from build123d import *

# Parameters (mm, degrees)
F1_DEPTH = 32
F2_R     = 6.5
F3_DEPTH = 25
F4_R     = 6.5
F5_DEPTH = 25
F6_R     = 6.5
F7_DEPTH = 25
F8_R     = 6.5
F9_DEPTH = 25


with BuildPart() as f1:
    # F0 (on Front) → F1 (new body)
    with BuildSketch(Plane.XZ):
        Polygon((0, 19.488953), (0, 0), (44, 0), (44, 17.170059), (69.764607, 17.170059), (69.764607, 0), (113, 0), (113, 18.089544), (88, 18.089544), (88, 64), (69, 64), (69, 30.170059), (44, 30.170059), (44, 64), (25, 64), (25, 19.488953), align=None)
    extrude(amount=F1_DEPTH)

    # F2 (on face) → F3 (cut)
    with BuildSketch(Plane.XY.offset(18.089544)):
        with Locations((99.580623, -15.326335)):
            Circle(F2_R)
    extrude(amount=-F3_DEPTH, mode=Mode.SUBTRACT)

    # F4 (on face) → F5 (cut)
    with BuildSketch(Plane.XY.offset(19.488953)):
        with Locations((12.18513, -16.29629)):
            Circle(F4_R)
    extrude(amount=-F5_DEPTH, mode=Mode.SUBTRACT)

    # F6 (on face) → F7 (cut)
    with BuildSketch(Plane.YZ.offset(88)):
        with Locations((-16.320663, 45.075346)):
            Circle(F6_R)
    extrude(amount=-F7_DEPTH, mode=Mode.SUBTRACT)

    # F8 (on face) → F9 (cut)
    with BuildSketch(Plane(origin=(25, 0, 0), x_dir=(0, -1, 0), z_dir=(-1, 0, 0))):
        with Locations((14.718622, 45.230217)):
            Circle(F8_R)
    extrude(amount=-F9_DEPTH, mode=Mode.SUBTRACT)


solid = f1.part
Design review of the part built by this model. Coordinates are the model's own, in mm. A direction names the side the tool comes from. Round coordinates to 2 decimals unless told otherwise and drop trailing zeros. Write each loop counter-clockwise with the first axis right and the second up, starting at its lowest first coordinate (ties: lowest second). Pieces come first, ordered by that corner, then holes. Notation, with made-up numbers: M 69.5,20.25 L 117.5,20.25 A18 cw 117.5,51.25 Z; hole C 42.25,-5 d6. An arc over 180 degrees is marked long. One line per item, written item: value. Start each with the question number.
1. Draft analysis for pull direction Y (two halves, no side actions). For faces 1 (the face through (56, -32, 25)), 2 (the face through (7.027, -20.251, 9.881)), 3 (the face through (57, -16, 30.17)), 4 (the face through (56, 0, 25)), state which applies: pulls with the +Y half, pulls with the -Y half, needs draft (parallel to the pull), parting line crosses it, or undercut.
2. To check wall thickness, follow probe 1 along X at (y, z) = (-6.5, 41); probe 2 along Y at (x, z) = (40.5, 45); probe 3 along Z at (x, y) = (108, -20). State the ranges of each line that lie inside material, in increasing order. Write a range as from..to.
3. Take a section at C-C on z = 9. State the section outline as (x, y) points, then the cut area to 3 significant figures.
4. Clearance check with flat-ended pins moving along their axes: P1, Ø12, axis at y = -19, z = 27, coming from the +X side; P2, Ø9.5, axis at y = -11, z = 46.5, coming from the -X side; P3, Ø7.5, axis at x = 95.5, y = -10, coming from the +Z side; P4, Ø10.5, axis at x = 12.19, y = -16.3, coming from the +Z side. State where each tip first meets the part, or that it passes through.
5. Take a section at B-B on z = 40.5. State the section outline as (x, y) points.
6. Take a section at D-D on x = 86.5. State the section outline as (y, z) points.
7. Take a section at A-A on y = -13. State how many separate pieces and enclosed holes the cut face has, then the cut area to 3 significant figures.
8. For faces 5 (the face through (69, -12, 51)), 6 (the face through (57, -16, 17.17)), 7 (the face through (25, -16, 37)), 8 (the face through (88, -16, 36)), list the 3-axis set-ups (+Z, -Z, +X, -X, +Y, -Y) from which the entire face can be reached by the end or side of a thin tool; tool diameter is ignored.
Computed:
1. face 1: pulls with the -Y half
1. face 2: undercut
1. face 3: needs draft
1. face 4: pulls with the +Y half
2. probe 1: x = 25..44, 69..88
2. probe 2: y = -32..-21.21, -8.22..0
2. probe 3: z = 0..18.09
3. outline: M 0,-32 L 44,-32 L 44,0 L 0,0 Z; M 69.76,-32 L 113,-32 L 113,0 L 69.76,0 Z; hole C 12.19,-16.3 d13; hole C 99.58,-15.33 d13
3. area: 2,530 mm²
4. P1: stops at x = 88
4. P2: stops at x = 25
4. P3: stops at z = 18.09
4. P4: passes through
5. outline: M 25,-32 L 44,-32 L 44,-19.18 L 25,-19.18 Z; M 25,-10.26 L 44,-10.26 L 44,0 L 25,0 Z; M 69,-32 L 88,-32 L 88,-20.94 L 69,-20.94 Z; M 69,-11.7 L 88,-11.7 L 88,0 L 69,0 Z
6. outline: M -32,0 L 0,0 L 0,64 L -32,64 Z; hole C -16.32,45.08 d13
7. separate pieces: 5
7. enclosed holes: 0
7. area: 2,790 mm²
8. face 5: +Z, +Y, -Y
8. face 6: -Z, +Y, -Y
8. face 7: +Z, -X, +Y, -Y
8. face 8: +Z, +X, +Y, -Y
